Verification items for the finished model (mm, model axes). A direction names the side the tool comes from. Round coordinates to 2 decimals unless told otherwise and drop trailing zeros. Write each loop counter-clockwise with the first axis right and the second up, starting at its lowest first coordinate (ties: lowest second). Pieces come first, ordered by that corner, then holes. Notation, with made-up numbers: M 53.25,35 L 111.25,35 A21 cw 111.25,64 Z; hole C 40.5,26 d10. An arc over 180 degrees is marked long. Answer in a Markdown table with one row per item. Add a question column.
1. Sectioned sample at C-C on x = -4.5. Record the cut outline in (y, z).
2. Sectioned sample at A-A on z = 3. Record the cut outline in (x, y), plus the area to 3 significant figures.
3. Draft check along X on faces 1 (the flat face through (0, 2.54, 37)), 2 (the cylindrical face through (-0.23, 1.25, 57.12)), 3 (the cylindrical face through (-0.29, 1.25, 64.12)). Enter one of: pulls with the +X half, pulls with the -X half, needs draft (parallel to the pull), parting line crosses it, or undercut.
4. Go/stop test with flat-tipped pins: pin 1 Ø14.5 at (x, z) = (0, 9.72) entering from +Y; pin 2 Ø1 at (y, z) = (0.5, 29.5) entering from -X; pin 3 Ø6 at (x, z) = (-15, 47.5) entering from -Y; pin 4 Ø3 at (y, z) = (-3.5, 20) entering from +X. Record where each tip stops, or that it passes through.
5. Sectioned sample at B-B on x = 0. Record the cut outline in (y, z), plus the area to 3 significant figures.
6. Sectioned sample at D-D on y = 1.25. Record the cut outline in (x, z).
7. Material ranges on probe 1 along Z at (x, y) = (0, 1); probe 2 along Z at (x, y) = (0, -3.4); probe 3 along Z at (x, y) = (0, -1.75), recorded low to high.
8. Set-up check for faces 4 (the flat face through (0, -3, 19)), 5 (the cylindrical face through (12.813, 1.288, 16.703)), 6 (the cylindrical face through (0.25, 1.25, 61.12)): record each of +Z, -Z, +X, -X, +Y, -Y from which the full face is reachable in a straight line by a thin tool's end or side.
```python
from build123d import *

# Parameters (mm, degrees)
SKETCH1_R           = 1.1
SKETCH1_R_2         = 8
BOSS_EXTRUDE1_DEPTH = 2.54
FILLET2_R           = 10
SKETCH1_4_R         = 8
SKETCH1_4_R_2       = 1.1
BOSS_EXTRUDE2_DEPTH = 2.999994
SKETCH2_R           = 9
SKETCH2_R_2         = 8
BOSS_EXTRUDE3_DEPTH = 1.27


with BuildPart() as part:
    # Sketch1 → Boss-Extrude1 (new body)
    with BuildSketch(Plane(origin=(0, 0, 0), x_dir=(1, 0, 0), z_dir=(0, 1, 0))):
        with BuildLine():
            Line((20.411129853, -60.145086441), (21.536156884, -59.674942586))
            Line((21.536156884, -59.674942586), (12.379162196, -16.260133485))
            ThreePointArc((12.379162196, -16.260133485), (0, 4.278699998), (-12.379162196, -16.260133485))
            Line((-12.379162196, -16.260133485), (-21.536156884, -59.674942586))
            Line((-21.536156884, -59.674942586), (-20.411129853, -60.145086441))
            ThreePointArc((-20.411129853, -60.145086441), (0, -64.119576268), (20.411129853, -60.145086441))
        make_face()
        with BuildLine():
            ThreePointArc((17.340734853, -58.106026106), (5.1e-08, -61.11957629), (-17.340734757, -58.10602614))
            ThreePointArc((-17.340734757, -58.10602614), (-18.548712659, -55.548529546), (-15.99121608, -54.340551611))
            ThreePointArc((-15.99121608, -54.340551611), (-6.8e-08, -57.119576403), (15.991215951, -54.340551657))
            ThreePointArc((15.991215951, -54.340551657), (18.548712618, -55.548529433), (17.340734853, -58.106026106))
        make_face(mode=Mode.SUBTRACT)
        with Locations((-11, -9.721300002)):
            Circle(SKETCH1_R, mode=Mode.SUBTRACT)
        with Locations((0, -9.721300002)):
            Circle(SKETCH1_R_2, mode=Mode.SUBTRACT)
        with Locations((0, 1.278699998)):
            Circle(SKETCH1_R, mode=Mode.SUBTRACT)
        with Locations((11, -9.721300002)):
            Circle(SKETCH1_R, mode=Mode.SUBTRACT)
    extrude(amount=BOSS_EXTRUDE1_DEPTH)

    # Fillet2
    fillet2_edges = [part.edges().sort_by_distance(p)[0] for p in [
        (12.379162196, 1.27, 16.260133485),
        (-12.379162196, 1.27, 16.260133485),
    ]]
    fillet(fillet2_edges, radius=FILLET2_R)

    # Sketch1_4 → Boss-Extrude2 (add)
    with BuildSketch(Plane(origin=(0, 0, 0), x_dir=(1, 0, 0), z_dir=(0, 1, 0))):
        with BuildLine():
            ThreePointArc((-12.379162196, -16.260133485), (0, -23.721300002), (12.379162196, -16.260133485))
            ThreePointArc((12.379162196, -16.260133485), (13.588750324, -13.089662308), (14, -9.721300002))
            ThreePointArc((14, -9.721300002), (-3.368362306, 3.867450323), (-12.379162196, -16.260133485))
        make_face()
        with BuildLine():
            ThreePointArc((-9.9, -9.721300002), (-10.307077747, -10.575617712), (-11.22701591, -10.797619553))
            ThreePointArc((-11.22701591, -10.797619553), (-11.692922253, -8.866982291), (-9.9, -9.721300002))
        make_face(mode=Mode.SUBTRACT)
        with Locations((0, -9.721300002)):
            Circle(SKETCH1_4_R, mode=Mode.SUBTRACT)
        with Locations((0, 1.278699998)):
            Circle(SKETCH1_4_R_2, mode=Mode.SUBTRACT)
        with BuildLine():
            ThreePointArc((12.1, -9.721300002), (11.854317711, -10.414222255), (11.22701591, -10.797619553))
            ThreePointArc((11.22701591, -10.797619553), (10.145682289, -9.028377748), (12.1, -9.721300002))
        make_face(mode=Mode.SUBTRACT)
    extrude(amount=-BOSS_EXTRUDE2_DEPTH)

    # Sketch2 → Boss-Extrude3 (add)
    with BuildSketch(Plane.XZ.offset(2.999994)):
        with Locations((0, 9.721300002)):
            Circle(SKETCH2_R)
        with Locations((0, 9.721300002)):
            Circle(SKETCH2_R_2, mode=Mode.SUBTRACT)
    extrude(amount=BOSS_EXTRUDE3_DEPTH)


solid = part.part
```
Geometry check:
| question | item | result |
|---|---|---|
| 1 | outline | M -4.27,1.93 L -3,1.93 L -3,-3.54 L 2.54,-3.54 L 2.54,3.11 L -4.27,3.11 Z; M -4.27,16.34 L 2.54,16.34 L 2.54,56.91 L 0,56.91 L 0,22.98 L -3,22.98 L -3,17.52 L -4.27,17.52 Z; M 0,60.92 L 2.54,60.92 L 2.54,63.93 L 0,63.93 Z |
| 2 | outline | M -12.28,-3 L -5.99,-3 L -5.99,-4.27 L -4.34,-4.27 L -4.34,2.54 L -12.28,2.54 Z; M 4.34,-4.27 L 5.99,-4.27 L 5.99,-3 L 12.28,-3 L 12.28,2.54 L 4.34,2.54 Z |
| 2 | area | 92.2 mm2 |
| 3 | face 1 | needs draft |
| 3 | face 2 | undercut |
| 3 | face 3 | parting line crosses it |
| 4 | pin 1 | passes through |
| 4 | pin 2 | stops at x = -15.28 |
| 4 | pin 3 | stops at y = 0 |
| 4 | pin 4 | stops at x = 10.84 |
| 5 | outline | M -4.27,0.72 L -3,0.72 L -3,-0.18 L 2.54,-0.18 L 2.54,1.72 L -4.27,1.72 Z; M -4.27,17.72 L 2.54,17.72 L 2.54,57.12 L 0,57.12 L 0,23.72 L -3,23.72 L -3,18.72 L -4.27,18.72 Z; M -3,-4.28 L 2.54,-4.28 L 2.54,-2.38 L -3,-2.38 Z; M 0,61.12 L 2.54,61.12 L 2.54,64.12 L 0,64.12 Z |
| 5 | area | 149 mm2 |
| 6 | outline | M -21.54,59.67 L -13.02,19.28 A10 cw -13.3,14.09 A14 ccw long 13.3,14.09 A10 cw 13.02,19.28 L 21.54,59.67 L 20.41,60.15 A54.4 ccw -20.41,60.15 Z; hole M -17.34,58.11 A2 ccw -15.99,54.34 A47.4 cw 15.99,54.34 A2 ccw 17.34,58.11 A51.4 ccw Z; hole C -11,9.72 d2.2; hole C 0,9.72 d16; hole C 0,-1.28 d2.2; hole C 11,9.72 d2.2 |
| 7 | probe 1 | z = -4.28 to -2.38, -0.18 to 1.72, 17.72 to 57.12, 61.12 to 64.12 |
| 7 | probe 2 | z = 0.72 to 1.72, 17.72 to 18.72 |
| 7 | probe 3 | z = -4.28 to -2.38, -0.18 to 1.72, 17.72 to 23.72 |
| 8 | face 4 | -Y |
| 8 | face 5 | +X, +Y, -Y |
| 8 | face 6 | +Y, -Y |
